Read the model definition and answer for the solid it produces. Units are mm, in the model's axes. A direction names the side the tool comes from. Give positions to 0.01 mm unless a question says otherwise; leave off trailing zeros. Loops run counter-clockwise (first coordinate to the right, second up) from the corner with the lowest first, then second, coordinate; pieces in that order, holes last. Notation, with made-up numbers: (64, 51) - (110, 51) arc R16 cw to (110, 82) - close; hole circle Ø10 at (17.25, -1). An arc over 180 degrees is marked (long way). Use a Markdown table: item, result. Add a question column.
Item 1: Consider probe 1 along X at (y, z) = (41, 15.25); probe 2 along X at (y, z) = (47, 2.5); probe 3 along Y at (x, z) = (18.45, 11) (3 decimals). Determine where each line is inside the solid, lowest interval first. Write a range as [from, to].
Item 2: A cutting plane is placed at D-D (z = 12.25). Give the number of separate pieces and of enclosed holes in the cut face, plus the area to 3 significant figures.
Item 3: Which of the six approach directions +Z, -Z, +X, -X, +Y, -Y give full straight-line access (tool end or side, diameter ignored) to faces 1 (the face through (14, 25, 15.25)), 2 (the face through (126, 45, 6.59)), 3 (the face through (12, 35, 11))?
Item 4: A cutting plane is placed at B-B (x = 82.5). Determine the outline of the cut face in (y, z), plus the area to 3 significant figures.
Item 5: A cutting plane is placed at C-C (z = 2.25). Determine the outline of the cut face in (x, y) (3 decimals).
Item 6: Each of these flat-tipped pins is pushed along its axis until it touches: P1, Ø4.5, axis at y = 24.875, z = 11, coming from the -X side; P2, Ø3, axis at y = 40.5, z = 9.5, coming from the +X side; P3, Ø10, axis at x = 33.5, y = 62.5, coming from the +Z side. Where does it stop, or does it pass through?
Item 7: A cutting plane is placed at A-A (y = 35). Determine the outline of the cut face in (x, z) (3 decimals), plus the area to 4 significant figures.
Item 8: For a pull along Y with two mould halves and no side action, classify faces 4 (the face through (140, 35, 2)), 5 (the face through (14, 45, 6.59)), 6 (the face through (15.9, 16.3, 4.9)) as +Y half, -Y half, draft (parallel to the pull), parting line (faces both ways), or undercut.
from build123d import *

# Parameters (mm, degrees)
SKETCH1_R           = 2.75
SKETCH1_W           = 100
SKETCH1_H           = 42.46
BOSS_EXTRUDE2_DEPTH = 4
SKETCH4_W           = 8
SKETCH4_H           = 42.46
BOSS_EXTRUDE3_DEPTH = 14
SKETCH5_R           = 4.125
CUT_EXTRUDE2_DEPTH  = 19
SKETCH7_R           = 2.75
CUT_EXTRUDE3_DEPTH  = 4
SKETCH8_R           = 2.75
CUT_EXTRUDE4_DEPTH  = 4
CUT_EXTRUDE8_DEPTH  = 4
CUT_EXTRUDE9_DEPTH  = 4
CUT_EXTRUDE12_DEPTH = 129


with BuildPart() as part:
    # Sketch1 → Boss-Extrude2 (new body)
    with BuildSketch(Plane.XY):
        with BuildLine():
            Line((140, 10.300871341), (140, 59.699128659))
            ThreePointArc((140, 59.699128659), (136.982944636, 66.982944636), (129.699128659, 70))
            Line((129.699128659, 70), (10.300871341, 70))
            ThreePointArc((10.300871341, 70), (3.017055364, 66.982944636), (0, 59.699128659))
            Line((0, 59.699128659), (0, 10.300871341))
            ThreePointArc((0, 10.300871341), (3.017055364, 3.017055364), (10.300871341, 0))
            Line((10.300871341, 0), (129.699128659, 0))
            ThreePointArc((129.699128659, 0), (136.982944636, 3.017055364), (140, 10.300871341))
        make_face()
        with Locations((10, 10)):
            Circle(SKETCH1_R, mode=Mode.SUBTRACT)
        with Locations((130, 10)):
            Circle(SKETCH1_R, mode=Mode.SUBTRACT)
        with Locations((10, 60)):
            Circle(SKETCH1_R, mode=Mode.SUBTRACT)
        with Locations((70, 35)):
            Rectangle(SKETCH1_W, SKETCH1_H, mode=Mode.SUBTRACT)
        with Locations((130, 60)):
            Circle(SKETCH1_R, mode=Mode.SUBTRACT)
    extrude(amount=BOSS_EXTRUDE2_DEPTH)

    # Sketch4 → Boss-Extrude3 (add)
    with BuildSketch(Plane.XY.offset(4)):
        with Locations((16, 35)):
            Rectangle(SKETCH4_W, SKETCH4_H)
        with Locations((124, 35)):
            Rectangle(SKETCH4_W, SKETCH4_H)
    extrude(amount=BOSS_EXTRUDE3_DEPTH)

    # Sketch5 → Cut-Extrude2 (cut, through all)
    with BuildSketch(Plane.XY.offset(18)):
        with Locations((20, 35)):
            Circle(SKETCH5_R)
        with Locations((120, 35)):
            Circle(SKETCH5_R)
    extrude(amount=-CUT_EXTRUDE2_DEPTH, mode=Mode.SUBTRACT)

    # Sketch7 → Cut-Extrude3 (cut)
    with BuildSketch(Plane(origin=(20, 0, 0), x_dir=(0, 0, -1), z_dir=(1, 0, 0))):
        with Locations((-11, 24.875)):
            Circle(SKETCH7_R)
        with Locations((-11, 45.125)):
            Circle(SKETCH7_R)
    extrude(amount=-CUT_EXTRUDE3_DEPTH, mode=Mode.SUBTRACT)

    # Sketch8 → Cut-Extrude4 (cut)
    with BuildSketch(Plane.ZY.offset(-120)):
        with Locations((11, 24.875)):
            Circle(SKETCH8_R)
        with Locations((11, 45.125)):
            Circle(SKETCH8_R)
    extrude(amount=-CUT_EXTRUDE4_DEPTH, mode=Mode.SUBTRACT)

    # Sketch12 → Cut-Extrude8 (cut)
    with BuildSketch(Plane.ZY.offset(-12)):
        Polygon((10.919872981, 19.875), (15.25, 22.375), (15.25, 27.375), (10.919872981, 29.875), (6.589745962, 27.375), (6.589745962, 22.375), align=None)
        Polygon((10.919872981, 40.125), (6.589745962, 42.625), (6.589745962, 47.625), (10.919872981, 50.125), (15.25, 47.625), (15.25, 42.625), align=None)
    extrude(amount=-CUT_EXTRUDE8_DEPTH, mode=Mode.SUBTRACT)

    # Sketch15 → Cut-Extrude9 (cut)
    with BuildSketch(Plane(origin=(128, 0, 0), x_dir=(0, 0, -1), z_dir=(1, 0, 0))):
        Polygon((-10.919872981, 19.875), (-15.25, 22.375), (-15.25, 27.375), (-10.919872981, 29.875), (-6.589745962, 27.375), (-6.589745962, 22.375), align=None)
        Polygon((-15.25, 47.625), (-15.25, 42.625), (-10.919872981, 40.125), (-6.589745962, 42.625), (-6.589745962, 47.625), (-10.919872981, 50.125), align=None)
    extrude(amount=-CUT_EXTRUDE9_DEPTH, mode=Mode.SUBTRACT)

    # Sketch16 → Cut-Extrude12 (cut, through all)
    with BuildSketch(Plane.ZY.offset(-12)):
        with BuildLine():
            Line((18, 13.77), (18, 23.236659765))
            ThreePointArc((18, 23.236659765), (17.110559955, 20.721820453), (14.837791617, 19.325380536))
            Line((14.837791617, 19.325380536), (7.162208383, 17.681279229))
            ThreePointArc((7.162208383, 17.681279229), (4.889440045, 16.284839312), (4, 13.77))
            Line((4, 13.77), (18, 13.77))
        make_face()
        with BuildLine():
            ThreePointArc((4, 56.23), (4.889440045, 53.715160688), (7.162208383, 52.318720771))
            Line((7.162208383, 52.318720771), (14.837791617, 50.674619464))
            ThreePointArc((14.837791617, 50.674619464), (17.110559955, 49.278179547), (18, 46.763340235))
            Line((18, 46.763340235), (18, 56.23))
            Line((18, 56.23), (4, 56.23))
        make_face()
    extrude(amount=-CUT_EXTRUDE12_DEPTH, mode=Mode.SUBTRACT)


solid = part.part
Geometry says:
| question | item | result |
|---|---|---|
| 1 | probe 1 | [12, 20], [120, 128] |
| 1 | probe 2 | [0, 20], [120, 140] |
| 1 | probe 3 | [18.503, 22.125], [27.625, 31.177], [38.823, 42.375], [47.875, 51.497] |
| 2 | separate pieces | 6 |
| 2 | enclosed holes | 0 |
| 2 | area | 252 mm² |
| 3 | face 1 | -X |
| 3 | face 2 | +X |
| 3 | face 3 | +Z, -X, +Y, -Y |
| 4 | outline | (0, 0) - (13.77, 0) - (13.77, 4) - (0, 4) - close; (56.23, 0) - (70, 0) - (70, 4) - (56.23, 4) - close |
| 4 | area | 110 mm² |
| 5 | outline | (0, 10.301) arc R10.301 ccw to (10.301, 0) - (129.699, 0) arc R10.301 ccw to (140, 10.301) - (140, 59.699) arc R10.301 ccw to (129.699, 70) - (10.301, 70) arc R10.301 ccw to (0, 59.699) - close; hole circle Ø5.5 at (10, 10); hole circle Ø5.5 at (10, 60); hole (20, 13.77) - (120, 13.77) - (120, 30.875) arc R4.125 ccw to (120, 39.125) - (120, 56.23) - (20, 56.23) - (20, 39.125) arc R4.125 ccw to (20, 30.875) - close; hole circle Ø5.5 at (130, 10); hole circle Ø5.5 at (130, 60) |
| 6 | P1 | through |
| 6 | P2 | x = 128 |
| 6 | P3 | z = 4 |
| 7 | outline | (0, 0) - (15.875, 0) - (15.875, 18) - (12, 18) - (12, 4) - (0, 4) - close; (124.125, 0) - (140, 0) - (140, 4) - (128, 4) - (128, 18) - (124.125, 18) - close |
| 7 | area | 235.5 mm² |
| 8 | face 4 | draft |
| 8 | face 5 | undercut |
| 8 | face 6 | -Y half |
